Input: dimensioned drawing with shaded views. Units: mm. Origin: part minimum x, y, z. Give positions to 0.01 mm unless a question says otherwise; leave off trailing zeros. Write each loop counter-clockwise with the first axis right and the second up, starting at its lowest first coordinate (ties: lowest second). Pieces come first, ordered by that corner, then holes. Notation, with made-up numbers: (-1.75, -10.75) -> (22.25, -10.75) arc R23 cw to (22.25, 3.25) -> close; hole circle Ø10 at (75, 58.25). An arc over 180 degrees is marked (long way). Return JSON: item names as keys, results as strings. Group by question number.
Item 1: Section C-C, the plane y = 0.95. Return loops of the section in (x, z), then the cut area to 3 significant figures.
Item 2: Section B-B, the plane x = 63.5. Return loops of the section in (y, z) (1 decimal).
Item 3: Section A-A, the plane z = 76.2. Return loops of the section in (x, y) (1 decimal).
Item 4: Line query: line 1 (Z direction, x = 63.5, y = 2.1); line 2 (Z direction, x = 12.7, y = 1.85); line 3 (X direction, y = 2.2, z = 80). Output: solid intervals per line, ascending. Write a range as [from, to].
Item 5: Section D-D, the plane x = 12.7. Return loops of the section in (y, z) (1 decimal), then the cut area to 3 significant figures.
Item 6: Pin query (flat end, axial travel): P1, Ø1.6, axis at x = 37, y = 2.5, coming from the +Z side; P2, Ø1.6, axis at y = 2, z = 68, coming from the -X side; P3, Ø1.5, axis at x = 31, y = 1, coming from the -Z side. Return the tip coordinate at first contact, or that it passes through.
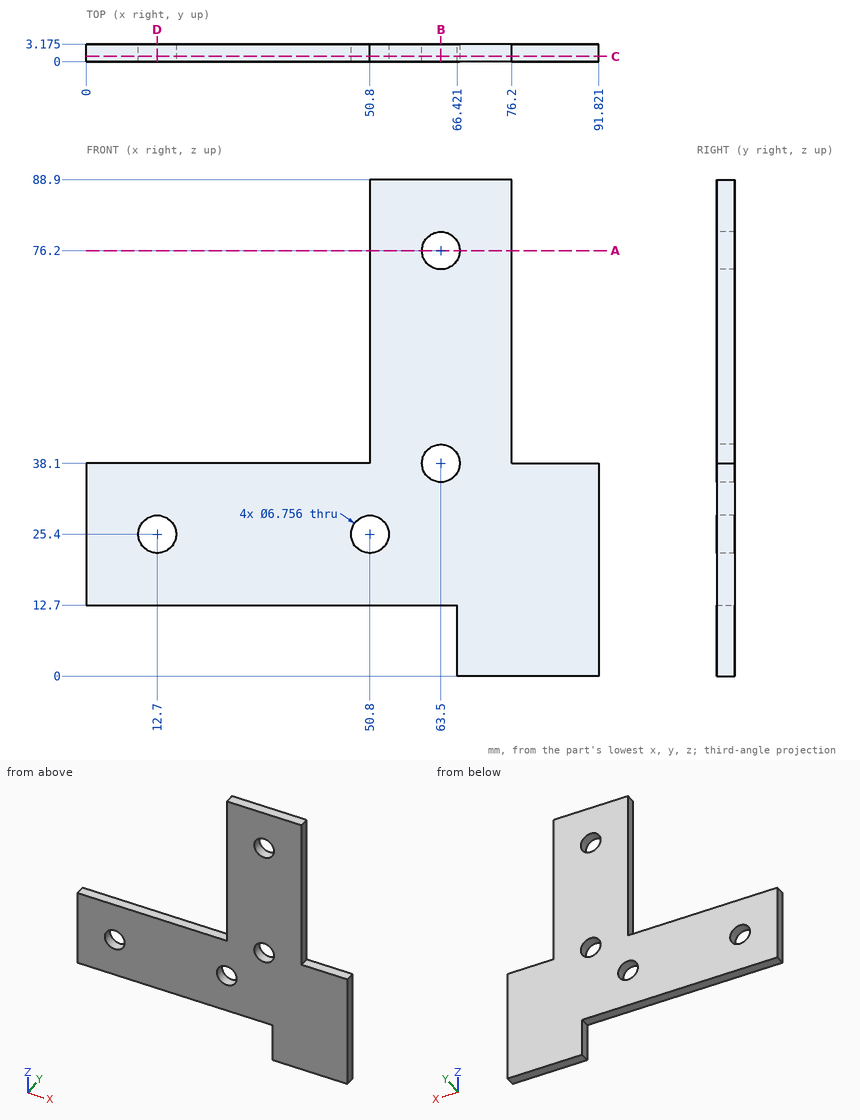
Answer below:
{
 "1": {"outline": "(0, 12.7) -> (66.42, 12.7) -> (66.42, 0) -> (91.82, 0) -> (91.82, 38.1) -> (76.2, 38.1) -> (76.2, 88.9) -> (50.8, 88.9) -> (50.8, 38.1) -> (0, 38.1) -> close; hole circle Ø6.76 at (12.7, 25.4); hole circle Ø6.76 at (50.8, 25.4); hole circle Ø6.76 at (63.5, 38.1); hole circle Ø6.76 at (63.5, 76.2)", "area": "3,800 mm2"},
 "2": {"outline": "(0, 12.7) -> (3.2, 12.7) -> (3.2, 34.7) -> (0, 34.7) -> close; (0, 41.5) -> (3.2, 41.5) -> (3.2, 72.8) -> (0, 72.8) -> close; (0, 79.6) -> (3.2, 79.6) -> (3.2, 88.9) -> (0, 88.9) -> close"},
 "3": {"outline": "(50.8, 0) -> (60.1, 0) -> (60.1, 3.2) -> (50.8, 3.2) -> close; (66.9, 0) -> (76.2, 0) -> (76.2, 3.2) -> (66.9, 3.2) -> close"},
 "4": {"line 1": "z = [12.7, 34.72], [41.48, 72.82], [79.58, 88.9]", "line 2": "z = [12.7, 22.02], [28.78, 38.1]", "line 3": "x = [50.8, 76.2]"},
 "5": {"outline": "(0, 12.7) -> (3.2, 12.7) -> (3.2, 22) -> (0, 22) -> close; (0, 28.8) -> (3.2, 28.8) -> (3.2, 38.1) -> (0, 38.1) -> close", "area": "59.2 mm2"},
 "6": {"P1": "stops at z = 38.1", "P2": "stops at x = 50.8", "P3": "stops at z = 12.7"}
}
